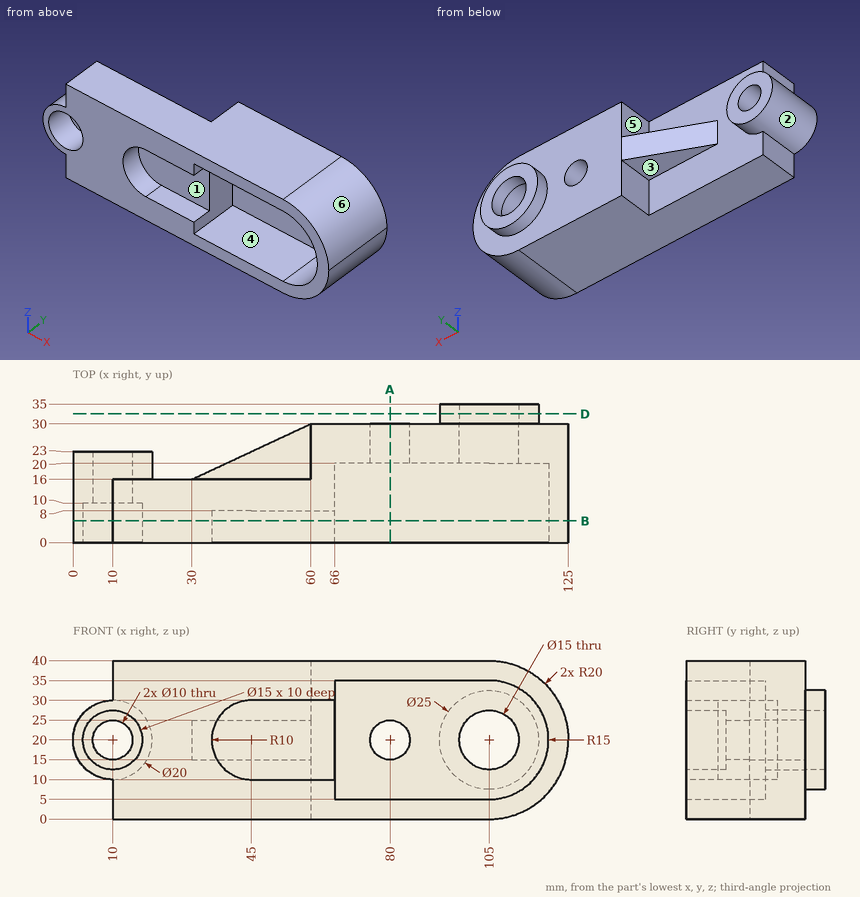
Part print with two shaded views. Sizes in mm from the minimum x, y, z corner. A direction names the side the tool comes from. Round coordinates to 2 decimals unless told otherwise and drop trailing zeros. Order: outer loops, then holes, each group sorted by start corner. A loop starts at its lowest first (then second) coordinate and runs counter-clockwise, first axis right, second up. Notation, with made-up numbers: M 44.25,37 L 65.25,37 A25 ccw 65.25,75 Z; hole C -36,12.5 d8. An arc over 180 degrees is marked long. Use CSV: the item, a comma, the result in double quotes. Start each with the question number.
(1) Cut at B-B on y = 5.5. State how many separate pieces and enclosed holes the cut face has, then the cut area to 3 significant figures.
(2) Drill centre lines: probe 1 along Z at (x, y) = (70, 9); probe 2 along X at (y, z) = (25.5, 20); probe 3 along X at (y, z) = (5.5, 15) (1 decimal). Where is each one in solid material? Low to high.
(3) Mould opens along Z. For the marked faces 4, 5 and 6 say: +Z half, -Z half, draft (parallel to the pull), parting line (faces both ways), or undercut.
(4) Cut at A-A on x = 80. List the corners of the cut face in (y, z).
(5) Tool access for the marked faces 1, 2 and 3: list every direction of +Z, -Z, +X, -X, +Y, -Y with a clear straight run to the whole face (end or side of a thin tool).
(6) Flat gauge pins, fed straight in: P1, Ø7, axis at x = 47, y = 25, coming from the +Z side; P2, Ø3, axis at y = 11.5, z = 3.5, coming from the -X side; P3, Ø6, axis at x = 45.5, z = 14, coming from the -Y side. Where does each tip first touch, or does it go through?
(7) Cut at D-D on y = 32.5. List the corners of the cut face in (x, z), then the cut area to 3 significant figures.
Findings:
1,separate pieces,"1"
1,enclosed holes,"2"
1,area,"2,310 mm^2"
2,probe 1,"z = 0 to 5, 35 to 40"
2,probe 2,"x = 50.36 to 75, 85 to 97.5, 112.5 to 125"
2,probe 3,"x = 1.3 to 4.4, 15.6 to 36.3, 119.1 to 124.4"
3,face 4,"undercut"
3,face 5,"draft"
3,face 6,"+Z half"
4,outline,"M 0,0 L 30,0 L 30,15 L 20,15 L 20,5 L 0,5 Z; M 0,35 L 20,35 L 20,25 L 30,25 L 30,40 L 0,40 Z"
5,face 1,"-Y"
5,face 2,"+Y"
5,face 3,"-Z, +Y"
6,P1,"stops at z = 25"
6,P2,"stops at x = 10"
6,P3,"stops at y = 8"
7,outline,"C 105,20 d25; hole C 105,20 d15"
7,area,"314 mm^2"
